Read the model definition and answer for the solid it produces. Units are mm, in the model's axes. Face numbers are marked on the shaded views. A direction names the side the tool comes from. Coordinates: 2 decimals unless noted, no trailing zeros. Order: outer loops, then holes, each group sorted by start corner. A loop starts at its lowest first (then second) coordinate and runs counter-clockwise, first axis right, second up. Notation, with made-up numbers: M -23.75,74.25 L -0.75,74.25 A4 ccw -0.75,78.25 Z; hole C -13,-32.75 d11. An arc over 180 degrees is marked long. Use a Markdown table: item, result. Add a question column.
1) Find section C-C on z = 9. Write down the section's boundary in (x, y).
2) Each of these flat-tipped pins is pushed along its axis until it touches: pin 1 Ø1 at (y, z) = (8.5, 8) entering from +X; pin 2 Ø14.5 at (y, z) = (15.5, 4) entering from -X; pin 3 Ø1.5 at (x, y) = (8, 8) entering from +Z; pin 4 Ø3 at (x, z) = (-3, 10) entering from +Y. Where does it stop, or does it pass through?
3) Find section B-B on y = 7.75. Write down the section's boundary in (x, z), plus the area to 3 significant figures.
4) For the marked faces 1, 2, 3 and 4, determine the directions among +Z, -Z, +X, -X, +Y, -Y from which every point of the face is accessible in a straight line to the end or side of a thin tool.
5) Find the intervals of material crossed by probe 1 along X at (y, z) = (21, 11.5); probe 2 along X at (y, z) = (14.25, 9); probe 3 along Y at (x, z) = (-16.5, -6.5), in increasing order. Write a range as [from, to].
6) The mould has two halves that part along X. Classify the marked faces 5, 6 and 7: released by +X, released by -X, zero draft, split by the parting line, or undercut.
7) Find section A-A on x = -20. Write down the section's boundary in (y, z).
8) Find section D-D on y = 11. Count the separate pieces of the cut face and the enclosed holes in it, plus the area to 3 significant figures.
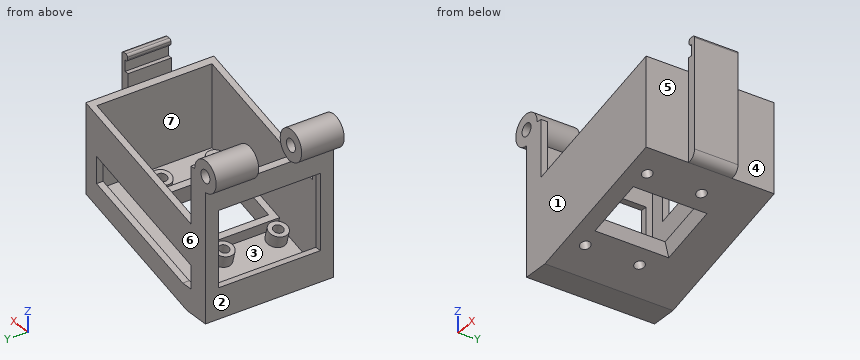
from build123d import *

# Parameters (mm, degrees)
BOSS_EXTRUDE1_DEPTH     = 29.5
SHELL1_T                = -1.5
SKETCH11_W              = 16
SKETCH11_H              = 20
BOSS_EXTRUDE6_DEPTH     = 2.75
CUT_EXTRUDE1_DEPTH      = 46.77263185
CUT_EXTRUDE1_DEPTH_BACK = 46.77263185
SKETCH3_W               = 13
SKETCH3_H               = 17
SKETCH4_R               = 2.125
BOSS_EXTRUDE2_DEPTH     = 2.8
SKETCH5_R               = 1.125
CUT_EXTRUDE2_DEPTH      = 44.905225798
SKETCH6_R               = 3.5
BOSS_EXTRUDE3_DEPTH     = 9.8
BOSS_EXTRUDE4_START     = -9.8
SKETCH7_R               = 3.5
BOSS_EXTRUDE4_DEPTH     = 9.8
SKETCH8_R               = 3.6
CUT_EXTRUDE3_DEPTH      = 9.9
SKETCH9_R               = 1.45
CUT_EXTRUDE4_DEPTH      = 44.135478309
SKETCH12_W              = 23
SKETCH12_H              = 10
BOSS_EXTRUDE7_DEPTH     = 1
SKETCH13_W              = 27
SKETCH13_H              = 10
BOSS_EXTRUDE8_DEPTH     = 1
SKETCH14_W              = 1.5
SKETCH14_H              = 10
BOSS_EXTRUDE9_DEPTH     = 0.8
FILLET2_R               = 0.5
FILLET3_R               = 0.5
FILLET4_R               = 2
CUT_EXTRUDE5_DEPTH      = 44.367750194
CUT_EXTRUDE6_REACH      = 56.452
SKETCH16_W              = 17
SKETCH16_H              = 23.5
CUT_EXTRUDE7_DEPTH      = 1.5


with BuildPart() as part:
    # Sketch2 → Boss-Extrude1 (new body)
    with BuildSketch(Plane(origin=(0, 0, 0), x_dir=(1, 0, 0), z_dir=(0, 1, 0))):
        Polygon((18.072476765, -16.342267954), (18.072476765, 6.657732046), (-14.927523235, 16.058029327), (-20.927523235, 16.058029327), (-20.927523235, -16.342267954), align=None)
    extrude(amount=BOSS_EXTRUDE1_DEPTH)

    # Shell1
    shell1_openings = [part.faces().sort_by_distance(p)[0] for p in [
        (-1.427523235, 14.75, 16.342267954),
    ]]
    offset(amount=SHELL1_T, openings=shell1_openings, kind=Kind.INTERSECTION)

    # Sketch11 → Boss-Extrude6 (add)
    with BuildSketch(Plane(origin=(2.699631824, 0, -9.477131153), x_dir=(0.9617413095492132, 0, 0.2739592186924259), z_dir=(-0.2739592186924259, 0, 0.9617413095492132))):
        with Locations((-0.825284328, 12.25)):
            Rectangle(SKETCH11_W, SKETCH11_H)
    extrude(amount=BOSS_EXTRUDE6_DEPTH)

    # Sketch3 → Cut-Extrude1 (cut, two sides: drawn at the far end of the back side and taken through both)
    with BuildSketch(Plane(origin=(2.699631824, 0, -9.477131153), x_dir=(0.9617413095492132, 0, 0.2739592186924259), z_dir=(-0.2739592186924259, 0, 0.9617413095492132)).offset(-CUT_EXTRUDE1_DEPTH_BACK)):
        with Locations((-0.825284328, 12.25)):
            Rectangle(SKETCH3_W, SKETCH3_H)
    extrude(amount=CUT_EXTRUDE1_DEPTH + CUT_EXTRUDE1_DEPTH_BACK, mode=Mode.SUBTRACT)

    # Sketch4 → Boss-Extrude2 (add)
    with BuildSketch(Plane(origin=(2.699631824, 0, -9.477131153), x_dir=(0.9617413095492132, 0, 0.2739592186924259), z_dir=(-0.2739592186924259, 0, 0.9617413095492132))):
        with Locations((9.674715672, 4.25)):
            Circle(SKETCH4_R)
        with Locations((9.674715672, 16.75)):
            Circle(SKETCH4_R)
        with Locations(Location((-11.325284328, 16.75, 0), (0, 0, 180))):
            Circle(SKETCH4_R)
        with Locations(Location((-11.325284328, 4.25, 0), (0, 0, 180))):
            Circle(SKETCH4_R)
    extrude(amount=BOSS_EXTRUDE2_DEPTH)

    # Sketch5 → Cut-Extrude2 (cut, through all)
    with BuildSketch(Plane(origin=(1.932546012, 0, -6.784255486), x_dir=(0.9617413095492132, 0, 0.2739592186924259), z_dir=(-0.2739592186924259, 0, 0.9617413095492132))):
        with Locations((9.674715672, 4.25)):
            Circle(SKETCH5_R)
        with Locations((9.674715672, 16.75)):
            Circle(SKETCH5_R)
        with Locations((-11.325284328, 4.25)):
            Circle(SKETCH5_R)
        with Locations((-11.325284328, 16.75)):
            Circle(SKETCH5_R)
    extrude(amount=-CUT_EXTRUDE2_DEPTH, mode=Mode.SUBTRACT)

    # Sketch6 → Boss-Extrude3 (add)
    with BuildSketch(Plane(origin=(0, 29.5, 0), x_dir=(1, 0, 0), z_dir=(0, 1, 0))):
        with Locations((-20.927523235, -16.342267954)):
            Circle(SKETCH6_R)
    extrude(amount=-BOSS_EXTRUDE3_DEPTH)

    # Sketch7 → Boss-Extrude4 (add)
    with BuildSketch(Plane(origin=(0, 0, 0), x_dir=(-1, 0, 0), z_dir=(0, -1, 0)).offset(BOSS_EXTRUDE4_START)):
        with Locations((20.927523235, -16.342267954)):
            Circle(SKETCH7_R)
    extrude(amount=BOSS_EXTRUDE4_DEPTH)

    # Sketch8 → Cut-Extrude3 (cut)
    with BuildSketch(Plane(origin=(0, 19.7, 0), x_dir=(-1, 0, 0), z_dir=(0, -1, 0))):
        with Locations((20.927523235, -16.342267954)):
            Circle(SKETCH8_R)
    extrude(amount=CUT_EXTRUDE3_DEPTH, mode=Mode.SUBTRACT)

    # Sketch9 → Cut-Extrude4 (cut, through all)
    with BuildSketch(Plane(origin=(0, 0, 0), x_dir=(-1, 0, 0), z_dir=(0, -1, 0))):
        with Locations(Location((20.927523235, -16.342267954, 0), (0, 0, 90))):
            Circle(SKETCH9_R)
    extrude(amount=-CUT_EXTRUDE4_DEPTH, mode=Mode.SUBTRACT)

    # Sketch12 → Boss-Extrude7 (add)
    with BuildSketch(Plane(origin=(18.072476765, 0, 0), x_dir=(0, 0, -1), z_dir=(1, 0, 0))):
        with Locations((-4.842267954, 14.75)):
            Rectangle(SKETCH12_W, SKETCH12_H)
    extrude(amount=BOSS_EXTRUDE7_DEPTH)

    # Sketch13 → Boss-Extrude8 (add)
    with BuildSketch(Plane(origin=(19.072476765, 0, 0), x_dir=(0, 0, -1), z_dir=(1, 0, 0))):
        with Locations((-6.842267954, 14.75)):
            Rectangle(SKETCH13_W, SKETCH13_H)
    extrude(amount=BOSS_EXTRUDE8_DEPTH)

    # Sketch14 → Boss-Extrude9 (add)
    with BuildSketch(Plane.ZY.offset(-19.072476765)):
        with Locations((19.592267954, 14.75)):
            Rectangle(SKETCH14_W, SKETCH14_H)
    extrude(amount=BOSS_EXTRUDE9_DEPTH)

    # Fillet2
    fillet2_edges = [part.edges().sort_by_distance(p)[0] for p in [
        (20.072476765, 14.75, 20.342267954),
        (18.272476765, 14.75, 18.842267954),
    ]]
    fillet(fillet2_edges, radius=FILLET2_R)

    # Fillet3
    fillet3_edges = [part.edges().sort_by_distance(p)[0] for p in [
        (18.272476765, 14.75, 20.342267954),
    ]]
    fillet(fillet3_edges, radius=FILLET3_R)

    # Fillet4
    fillet4_edges = [part.edges().sort_by_distance(p)[0] for p in [
        (20.072476765, 14.75, -6.657732046),
    ]]
    fillet(fillet4_edges, radius=FILLET4_R - 0.0001)  # a hair under: the kernel refuses the full size

    # Sketch15 → Cut-Extrude5 (cut, through all)
    with BuildSketch(Plane(origin=(0, 29.5, 0), x_dir=(1, 0, 0), z_dir=(0, 1, 0))):
        Polygon((18.072476765, -13.342267954), (-16.247523235, -3.565958782), (-16.247523235, -6.478203224), (-16.247523235, -16.342267954), (18.072476765, -16.342267954), align=None)
    extrude(amount=-CUT_EXTRUDE5_DEPTH, mode=Mode.SUBTRACT)

    # Sketch16 → Cut-Extrude6 (cut, up to next)
    with BuildSketch(Plane.ZY.offset(20.927523235), mode=Mode.PRIVATE) as cut_extrude6_sk1:
        with Locations((-0.657732046, 14.75)):
            Rectangle(SKETCH16_W, SKETCH16_H)
    cut_extrude6_tool1 = extrude(cut_extrude6_sk1.sketch, amount=-CUT_EXTRUDE6_REACH, mode=Mode.PRIVATE) & part.part
    add(cut_extrude6_tool1.solids().sort_by_distance((-20.927523, 14.75, -0.657732))[0], mode=Mode.SUBTRACT)

    # Sketch17 → Cut-Extrude7 (cut)
    with BuildSketch(Plane(origin=(0, 29.5, 0), x_dir=(1, 0, 0), z_dir=(0, 1, 0))):
        Polygon((-16.247523235, 5.483028504), (14.579138142, -3.298176984), (14.579138142, 2.701823016), (-13.521396163, 10.70647078), (-16.247523235, 10.70647078), align=None)
    extrude(amount=-CUT_EXTRUDE7_DEPTH, mode=Mode.SUBTRACT)


solid = part.part
Check result:
| question | item | result |
|---|---|---|
| 1 | outline | M -20.93,0 L -16.25,0 L -16.25,1.5 L -19.43,1.5 L -19.43,28 L -16.25,28 L -16.25,29.5 L -20.93,29.5 Z; M 2.83,0 L 18.07,0 L 18.07,9.75 L 20.07,9.75 L 20.07,19.75 L 18.07,19.75 L 18.07,29.5 L 2.83,29.5 L 2.83,28 L 16.57,28 L 16.57,1.5 L 2.83,1.5 Z |
| 2 | pin 1 | stops at x = 18.07 |
| 2 | pin 2 | stops at x = -20.93 |
| 2 | pin 3 | stops at z = -4.89 |
| 2 | pin 4 | passes through |
| 3 | outline | M -20.93,-16.06 L -14.93,-16.06 L -3.93,-12.93 L -5.1,-8.84 L -6.54,-9.25 L -5.79,-11.89 L -15.14,-14.56 L -19.43,-14.56 L -19.43,-9.16 L -20.93,-9.16 Z; M -20.93,7.84 L -19.43,7.84 L -19.43,13.18 A3.5 ccw long -20.93,12.84 Z; M 7.4,-5.28 L 8.57,-9.37 L 18.07,-6.66 L 18.07,13.34 L 16.57,12.91 L 16.57,-5.53 L 9.6,-7.51 L 8.85,-4.87 Z; hole C -20.93,16.34 d2.9 |
| 3 | area | 125 mm2 |
| 4 | face 1 | +Z, -Z, +X, -X, -Y |
| 4 | face 2 | -Z, -X, +Y, -Y |
| 4 | face 3 | none |
| 4 | face 4 | +Z, -Z, +X, +Y |
| 5 | probe 1 | x = [-20.93, -19.43], [16.57, 18.07] |
| 5 | probe 2 | x = [-20.93, -19.43], [16.57, 20.07] |
| 5 | probe 3 | y = [0, 1.5], [28, 29.5] |
| 6 | face 5 | released by +X |
| 6 | face 6 | zero draft |
| 6 | face 7 | undercut |
| 7 | outline | M 0,-16.06 L 29.5,-16.06 L 29.5,15.23 L 19.7,15.23 L 19.7,12.86 L 9.8,12.86 L 9.8,15.23 L 0,15.23 Z; M 0,17.46 L 9.8,17.46 L 9.8,19.72 L 0,19.72 Z; M 19.7,17.46 L 29.5,17.46 L 29.5,19.72 L 19.7,19.72 Z; hole M 3,-9.16 L 26.5,-9.16 L 26.5,7.84 L 3,7.84 Z |
| 8 | separate pieces | 3 |
| 8 | enclosed holes | 0 |
| 8 | area | 143 mm2 |
